from build123d import *

# Parameters (mm, degrees)
F1_DEPTH = 660.4
F2_W     = 584.2
F2_H     = 173.0248
F3_DEPTH = 355.601
F5_DEPTH = 25.4
F7_D     = 6.35


with BuildPart() as f1:
    # F0 (on Right) → F1 (new body)
    with BuildSketch(Plane.YZ):
        Polygon((-188.84479, 4.7752), (-188.84479, 0), (166.75521, 0), (166.75521, 203.2), (161.98001, 203.2), (161.98001, 4.7752), align=None)
    extrude(amount=F1_DEPTH)

    # F2 (on face) → F3 (cut, through all)
    with BuildSketch(Plane.XZ.offset(188.84479)):
        with Locations((330.2, 91.2876)):
            Rectangle(F2_W, F2_H)
    extrude(amount=-F3_DEPTH, mode=Mode.SUBTRACT)

    # F4 (on face) → F5 (cut)
    with BuildSketch(Plane.XY.offset(4.7752)):
        Polygon((622.3, 166.75521), (38.1, 166.75521), (38.1, 161.98001), (38.1, -148.16235), (622.3, -148.16235), align=None)
    extrude(amount=-F5_DEPTH, mode=Mode.SUBTRACT)

    # F7 (through all)
    with Locations(Plane.XZ.offset(-161.98001)):
        with Locations((19.05, 190.5), (38.1, 190.5), (57.15, 190.5), (76.2, 190.5), (95.25, 190.5), (114.3, 190.5), (133.35, 190.5), (152.4, 190.5), (171.45, 190.5), (190.5, 190.5), (209.55, 190.5), (228.6, 190.5), (247.65, 190.5), (266.954, 190.5), (286.004, 190.5), (305.054, 190.5), (324.358, 190.5), (343.408, 190.5), (362.458, 190.5), (381.508, 190.5), (400.812, 190.5), (420.116, 190.5), (439.166, 190.5), (458.216, 190.5), (477.266, 190.5), (496.57, 190.5), (515.874, 190.5), (534.924, 190.5), (553.974, 190.5), (573.024, 190.5), (611.124, 190.5), (592.074, 190.5), (641.35, 190.5)):
            Hole(F7_D / 2)


solid = f1.part
Geometry: final body of the model. Coordinates: model frame, mm. A direction names the side the tool comes from. Give positions to 0.01 mm unless a question says otherwise; leave off trailing zeros. Write each loop counter-clockwise with the first axis right and the second up, starting at its lowest first coordinate (ties: lowest second). Pieces come first, ordered by that corner, then holes. Notation, with made-up numbers: (77, -18) -> (107, -18) arc R23 cw to (107, 15) -> close; hole circle Ø2 at (87.5, 47.5). An arc over 180 degrees is marked (long way). Answer as a JSON object with one key per item and string values.
1. Ray query, probe 1 along Z at (x, y) = (114.3, 164.15) (3 decimals); probe 2 along Z at (x, y) = (250, -154). Return the intervals inside material, ascending. Write a range as from..to.
Ans:
{"probe 1": "z = 177.8..187.325, 193.675..203.2", "probe 2": "z = 0..4.78"}
2. Contact query for flat-ended pins moving along their axis: pin 1 (5 mm diameter, centred on x = 592.074, z = 190.5, fed in from -Y); pin 2 (4 mm diameter, centred on x = 401.5, z = 1.5, fed in from +Y); pin 3 (10 mm diameter, centred on x = 114.3, z = 190.5, fed in from -Y). Output: stop coordinate, or through.
Ans:
{"pin 1": "passes through", "pin 2": "stops at y = -148.16", "pin 3": "stops at y = 161.98"}
3. Cut plane B-B on z = 42.5. Output: boundary loops of the cut face in (x, y).
Ans:
{"outline": "(0, 161.98) -> (38.1, 161.98) -> (38.1, 166.76) -> (0, 166.76) -> close; (622.3, 161.98) -> (660.4, 161.98) -> (660.4, 166.76) -> (622.3, 166.76) -> close"}
4. Access query for faces 1 (the flat face through (660.4, -12, 4)), 2 (the flat face through (304, 161.98, 178)). Directions: +Z, -Z, +X, -X, +Y, -Y. A direction counts if a zero-diameter tool reaches every point of the face in a straight line with its end or side. Return the directions, or none.
Ans:
{"face 1": "+Z, -Z, +X, +Y, -Y", "face 2": "+Z, +X, -X, -Y"}
5. Cut plane A-A on y = 89.5. Output: boundary loops of the cut face in (x, z), and give its area (3 significant figures).
Ans:
{"outline": "(0, 0) -> (38.1, 0) -> (38.1, 4.78) -> (0, 4.78) -> close; (622.3, 0) -> (660.4, 0) -> (660.4, 4.78) -> (622.3, 4.78) -> close", "area": "364 mm^2"}
